The figure shows three views and two pictorial views of one solid part (mm, origin at its lowest corner). Answer the questions. Give positions to 0.01 mm unless a question says otherwise; leave off trailing zeros. Loops run counter-clockwise (first coordinate to the right, second up) from the corner with the lowest first, then second, coordinate; pieces in that order, holes last. Notation, with made-up numbers: (74, 33.5) - (91, 33.5) arc R16 ccw to (91, 38.5) - close; hole circle Ø5 at (14.25, -20). An arc over 180 degrees is marked (long way). Use a Markdown table: item, result. Add a question column.
Item 1: Consider probe 1 along X at (y, z) = (2.5, 18.5) (1 decimal); probe 2 along Y at (x, z) = (3.5, 18); probe 3 along Y at (x, z) = (1.5, 10) (1 decimal). Determine where each line is inside the solid, lowest interval first. Write a range as [from, to].
Item 2: A cutting plane is placed at C-C (z = 30). Determine the outline of the cut face in (x, y).
Item 3: A cutting plane is placed at D-D (y = 6.25). Determine the outline of the cut face in (x, z).
Item 4: A cutting plane is placed at A-A (y = 3.5). Determine the outline of the cut face in (x, z).
Item 5: A cutting plane is placed at B-B (x = 4.5). Determine the outline of the cut face in (y, z) (1 decimal).
Item 6: Each of these flat-tipped pins is pushed along its axis until it touches: P1, Ø1.5, axis at x = 5.5, z = 27, coming from the -Y side; P2, Ø1, axis at x = 1, z = 12.5, coming from the -Y side; P3, Ø2, axis at x = 5, z = 26, coming from the +Y side. Where does it stop, or does it pass through?
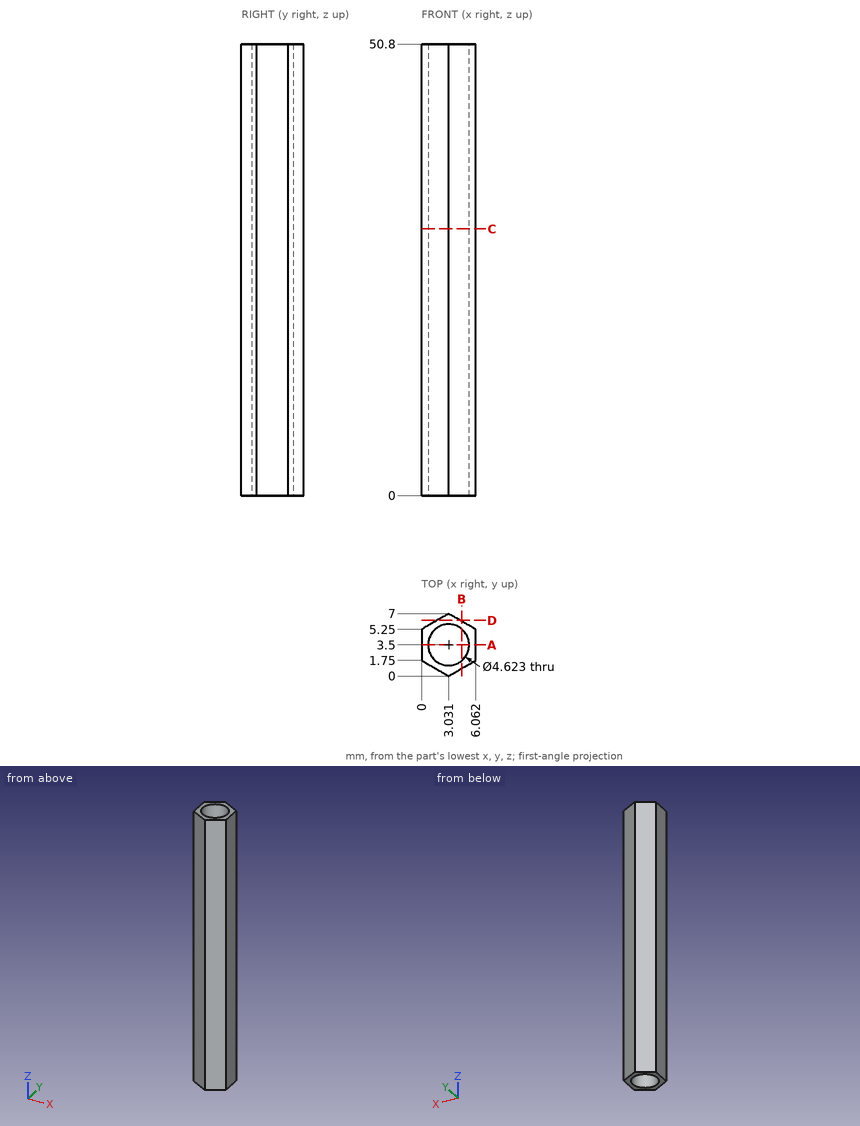
Geometry says:
| question | item | result |
|---|---|---|
| 1 | probe 1 | [0, 0.9], [5.1, 6.1] |
| 1 | probe 2 | [0.27, 1.24], [5.76, 6.73] |
| 1 | probe 3 | [0.9, 1.8], [5.2, 6.1] |
| 2 | outline | (0, 1.75) - (3.03, 0) - (6.06, 1.75) - (6.06, 5.25) - (3.03, 7) - (0, 5.25) - close; hole circle Ø4.62 at (3.03, 3.5) |
| 3 | outline | (1.73, 0) - (4.33, 0) - (4.33, 50.8) - (1.73, 50.8) - close |
| 4 | outline | (0, 0) - (0.72, 0) - (0.72, 50.8) - (0, 50.8) - close; (5.34, 0) - (6.06, 0) - (6.06, 50.8) - (5.34, 50.8) - close |
| 5 | outline | (0.8, 0) - (1.7, 0) - (1.7, 50.8) - (0.8, 50.8) - close; (5.3, 0) - (6.2, 0) - (6.2, 50.8) - (5.3, 50.8) - close |
| 6 | P1 | y = 0.99 |
| 6 | P2 | y = 0.88 |
| 6 | P3 | y = 6.44 |
